Autodesk Inventor part; units mm, degrees
ref_plane "YZ Plane" through (0, 0, 0) normal (1, 0, 0) x (0, 1, 0)
ref_plane "XZ Plane" through (0, 0, 0) normal (0, 1, 0) x (-1, 0, 0)
ref_plane "XY Plane" through (0, 0, 0) normal (0, 0, 1) x (1, 0, 0)
sketch "スケッチ1" plane through (0, 0, 0) normal (1, 0, 0) x (0, 1, 0)
  line L0 (0, 0) -> (15, 0)
  line L1 (15, 0) -> (15, -16)
  line L2 (15, -16) -> (0, -16)
  line L3 (0, -16) -> (0, 0)
  circle A0 centre (4, -20) radius 4
  circle A1 centre (4, -20) radius 1.6
  line L4 (15, -16) -> (6.5693, -23.0657)
  line L5 (0, -20) -> (0, -16)
  dimension "d0" = 15
  dimension "d2" = 3.2
  dimension "d3" = 8
  dimension "d5" = 20
extrude "プレート1" add sketch "スケッチ1" along normal blind 1.5
sketch "スケッチ2" plane through (1.5, 0, 0) normal (1, 0, 0) x (0, 0, -1)
  circle A0 centre (2, 10) radius 0.8
  circle A1 centre (2, 2) radius 0.8
  circle A2 centre (20, 4) radius 1.6
  line L0 (0, 15) -> (16, 15)
  line L1 (0, 0) -> (0, 15)
  line L2 (20, 0) -> (0, 0)
  arc A3 (20, 0) -> (23.0657, 6.5693) centre (20, 4) ccw
  line L3 (16, 15) -> (23.0657, 6.5693)
  circle A4 centre (14, 2) radius 0.8
  line L4 (5, 13) -> (16, 13)
  line L5 (16, 13) -> (16, 5)
  line L6 (16, 5) -> (5, 5)
  line L7 (5, 5) -> (5, 13)
  dimension "d8" = 2
  dimension "d9" = 3
  dimension "d10" = 3
extrude "切り取り1" cut sketch "スケッチ2" against normal blind 1.5 contours A0 | A1 | A4 | L4 L5 L6 L7
equation "\"d6\" = Thickness"
equation "\"d4\" = Thickness"
equation "\"BendRadius\" = Thickness"
equation "\"BendReliefWidth\" = Thickness"
equation "\"BendReliefDepth\" = 0.5 * Thickness"
equation "\"CornerReliefSize\" = 4 * Thickness"
equation "\"MinimumRemnant\" = 2 * Thickness"
equation "\"TransitionRadius\" = BendRadius"
equation "\"JacobiRadiusSize\" = BendRadius"
equation "\"GapSize\" = Thickness"
properties part number "battery_cover_setter_joint"
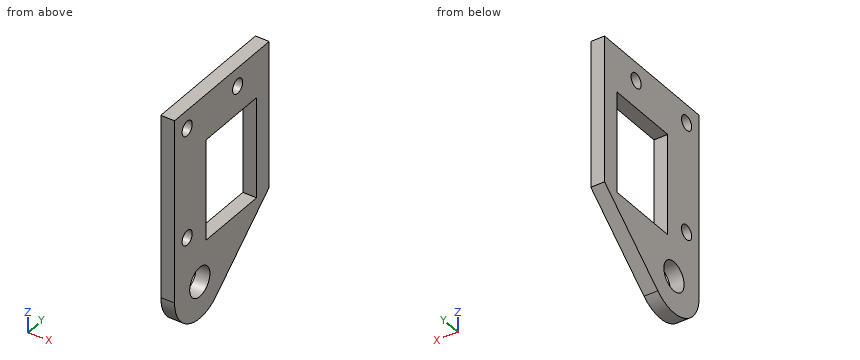
Design review of the part built by this model. Coordinates are the model's own, in mm. Round coordinates to 2 decimals unless told otherwise and drop trailing zeros. Order: outer loops, then holes, each group sorted by start corner. A loop starts at its lowest first (then second) coordinate and runs counter-clockwise, first axis right, second up. Notation, with made-up numbers: (81, -10.5) - (87, -10.5) arc R6 cw to (87, -3.5) - close; hole circle Ø1 at (50.5, -6.75). An arc over 180 degrees is marked (long way). One line per question, with ' | ' between items.
Item 1: For P1, Ø0.8, axis at x = 0.5, y = 7, coming from the -Z side, flat-tipped, find the tip position at first contact; note if it passes through.
Checks:
P1: z = -23.04
Item 2: Wall thickness on line 1 (Y direction, x = 0.95, z = -2); line 2 (Z direction, x = 0.75, y = 4); line 3 (Y direction, x = 0.7, z = -15.25): over which ranges is each line inside the solid? List them lowest first. Write a range as [from, to].
Checks:
line 1: [0, 1.2], [2.8, 9.2], [10.8, 15] | line 2: [-24, -21.6], [-18.4, 0] | line 3: [0, 5], [13, 15]
Item 3: Take a section at D-D, the plane y = 2. Write out the cut boundary in (x, z).
Checks:
outline: (0, -23.46) - (1.5, -23.46) - (1.5, -14.8) - (0, -14.8) - close; (0, -13.2) - (1.5, -13.2) - (1.5, -2.8) - (0, -2.8) - close; (0, -1.2) - (1.5, -1.2) - (1.5, 0) - (0, 0) - close
Item 4: Take a section at A-A, the plane z = -2. Write out the cut boundary in (x, y).
Checks:
outline: (0, 0) - (1.5, 0) - (1.5, 1.2) - (0, 1.2) - close; (0, 2.8) - (1.5, 2.8) - (1.5, 9.2) - (0, 9.2) - close; (0, 10.8) - (1.5, 10.8) - (1.5, 15) - (0, 15) - close
Item 5: Take a section at C-C, the plane z = -11.75. Write out the cut boundary in (x, y).
Checks:
outline: (0, 0) - (1.5, 0) - (1.5, 5) - (0, 5) - close; (0, 13) - (1.5, 13) - (1.5, 15) - (0, 15) - close
Item 6: Take a section at B-B, the plane x = 1. Write out the cut boundary in (y, z).
Checks:
outline: (0, -20) arc R4 ccw to (6.57, -23.07) - (15, -16) - (15, 0) - (0, 0) - close; hole circle Ø1.6 at (2, -14); hole circle Ø1.6 at (2, -2); hole circle Ø3.2 at (4, -20); hole (5, -16) - (13, -16) - (13, -5) - (5, -5) - close; hole circle Ø1.6 at (10, -2)
